```python
from build123d import *

# Parameters (mm, degrees)
SKETCH2_R          = 4
CUT_EXTRUDE1_DEPTH = 30


with BuildPart() as part:
    # Sketch1 → Revolve1 (revolve)
    with BuildSketch(Plane(origin=(0, 0, 0), x_dir=(0, 0, -1), z_dir=(1, 0, 0))):
        Polygon((0, 0), (50, 0), (50, 70), (55, 70), (55, 75), (0, 75), align=None)
    revolve(axis=Axis((0, 75, 0), (0, -1, 0)))

    # Sketch2 → Cut-Extrude1 (cut)
    with BuildSketch(Plane.XZ):
        with Locations((-24.748737342, 24.748737342)):
            Circle(SKETCH2_R)
        with Locations((24.748737342, 24.748737342)):
            Circle(SKETCH2_R)
        with Locations((24.748737342, -24.748737342)):
            Circle(SKETCH2_R)
        with Locations((-24.748737342, -24.748737342)):
            Circle(SKETCH2_R)
    extrude(amount=-CUT_EXTRUDE1_DEPTH, mode=Mode.SUBTRACT)


solid = part.part
```
Source: CAD feature listing. Evaluate the final solid. Frame: model axes, mm. A direction names the side the tool comes from. Coordinates: 2 decimals unless noted, no trailing zeros. Loops run counter-clockwise (first coordinate to the right, second up) from the corner with the lowest first, then second, coordinate; pieces in that order, holes last. Notation, with made-up numbers: M 39,54.25 L 43,54.25 A18 cw 43,79.25 Z; hole C -16.5,-24.5 d7. An arc over 180 degrees is marked long. Put each result on its own line as item: value. Start each with the question number.
1) Cut plane D-D on y = 50.5. Return the cut outline in (x, z), then the cut area to 3 significant figures.
2) Pull-direction query (Z, two-part tool) for faces 3 (the face through (25, 30, 25)), 4 (the face through (-49, 70, 12)), 5 (the face through (15.02, 35.49, -47.69)); classes: pulls with the +Z half, pulls with the -Z half, needs draft (parallel to the pull), parting line crosses it, or undercut.
3) Contact query for flat-ended pins moving along their axis: pin 1 Ø10 at (x, y) = (22.5, 32) entering from +Z; pin 2 Ø2 at (x, y) = (-12, 13.5) entering from -Z (3 decimals); pin 3 Ø12 at (y, z) = (34, -30.5) entering from -X. Output: stop coordinate, or through.
4) Cut plane C-C on y = 9.5. Return the cut outline in (x, z), then the cut area to 3 significant figures.
5) Reachability of faces 1 (the face through (1, 0, -1)), 2 (the face through (-25.616, 14.79, 20.844)) from +Z, -Z, +X, -X, +Y, -Y: full face, straight path, thin tool, end or side. Return the list, or none.
6) Cut plane B-B on x = 0. Return the cut outline in (y, z).
7) Ray query, L1, parallel to X at y = 18, z = -25.5; L2, parallel to Z at x = 27, y = 11.5; L3, parallel to Y at x = -5.5, z = -50. Return the intervals inside material, ascending. Write a range as from..to.
8) Cut plane A-A on z = 0. Return the cut outline in (x, y).
The answers:
1. outline: C 0,0 d100
1. area: 7,850 mm²
2. face 3: undercut
2. face 4: needs draft
2. face 5: parting line crosses it
3. pin 1: stops at z = 46.84
3. pin 2: stops at z = -48.775
3. pin 3: stops at x = -43.59
4. outline: C 0,0 d100; hole C -24.75,-24.75 d8; hole C -24.75,24.75 d8; hole C 24.75,-24.75 d8; hole C 24.75,24.75 d8
4. area: 7,650 mm²
5. face 1: +Z, -Z, +X, -X, -Y
5. face 2: -Y
6. outline: M 0,-50 L 70,-50 L 70,-55 L 75,-55 L 75,55 L 70,55 L 70,50 L 0,50 Z
7. L1: x = -43.01..-28.68, -20.82..20.82, 28.68..43.01
7. L2: z = -42.08..-28.06, -21.44..21.44, 28.06..42.08
7. L3: y = 70..75
8. outline: M -55,70 L -50,70 L -50,0 L 50,0 L 50,70 L 55,70 L 55,75 L -55,75 Z
